Can you work these out from the model? Positions are in its coordinate system, mm. A direction names the side the tool comes from. Round coordinates to 2 decimals unless told otherwise and drop trailing zeros. Order: outer loops, then holes, each group sorted by start corner. A loop starts at its lowest first (then second) coordinate and runs counter-clockwise, first axis right, second up. Notation, with made-up numbers: (72, 6) -> (84, 6) arc R24 ccw to (84, 27) -> close; hole circle Ø7 at (-9.5, -12.5). An arc over 180 degrees is marked (long way). One line per item, written item: value.
```python
from build123d import *

# Parameters (mm, degrees)
F1_R     = 3
F2_DEPTH = 25
F0_R     = 4
F3_DEPTH = 14
F4_R     = 4
F4_R_2   = 3
F5_DEPTH = 11
F7_D     = 4


with BuildPart() as f2:
    # F1 (on Front) → F2 (new body)
    with BuildSketch(Plane.XZ):
        Circle(F1_R)
    extrude(amount=F2_DEPTH)

    # F0 (on Front) → F3 (join)
    with BuildSketch(Plane.XZ):
        Circle(F0_R)
    extrude(amount=F3_DEPTH)

    # F4 (on face) → F5 (cut)
    with BuildSketch(Plane(origin=(0, 0, 0), x_dir=(-1, 0, 0), z_dir=(0, 1, 0))):
        Circle(F4_R)
        Circle(F4_R_2, mode=Mode.SUBTRACT)
    extrude(amount=-F5_DEPTH, mode=Mode.SUBTRACT)

    # F7 (through all)
    with Locations(Plane(origin=(0, 0, 0), x_dir=(-1, 0, 0), z_dir=(0, 1, 0))):
        with Locations((0, 0)):
            Hole(F7_D / 2)


solid = f2.part
```
Q1. I want a section at A-A on x = 0. List the corners of the cut face in (y, z) for me.
Answers below:
outline: (-25, -3) -> (-14, -3) -> (-14, -4) -> (-11, -4) -> (-11, -3) -> (0, -3) -> (0, -2) -> (-25, -2) -> close; (-25, 2) -> (0, 2) -> (0, 3) -> (-11, 3) -> (-11, 4) -> (-14, 4) -> (-14, 3) -> (-25, 3) -> close
Q2. On a 3-axis mill with a long thin cutter (end or side, diameter ignored), from which of +Z, -Z, +X, -X, +Y, -Y can I reach the whole of each face in a straight line? I mean faces 4 (the face through (-1, -11, 3)), 5 (the face through (1, -25, -2)). Say none if no direction works.
Answers below:
face 4: +Y
face 5: +Z, -Z, +X, -X, -Y
Q3. I want a section at B-B on z = 0. List the corners of the cut face in (x, y) for me.
Answers below:
outline: (-4, -14) -> (-3, -14) -> (-3, -25) -> (-2, -25) -> (-2, 0) -> (-3, 0) -> (-3, -11) -> (-4, -11) -> close; (2, -25) -> (3, -25) -> (3, -14) -> (4, -14) -> (4, -11) -> (3, -11) -> (3, 0) -> (2, 0) -> close
Q4. I want a section at C-C on y = -6. List the corners of the cut face in (x, z) for me.
Answers below:
outline: circle Ø6 at (0, 0); hole circle Ø4 at (0, 0)
Q5. Will these pins go through, and if not, where does the flat tip stop? pin 1 Ø1 at (x, y) = (-1.5, -12) entering from +Z; pin 2 Ø3 at (x, z) = (0, 0) entering from -Y; pin 3 Ø1 at (x, y) = (3, -21.5) entering from +Z; pin 4 Ø1 at (x, y) = (1.5, -21) entering from -Z.
Answers below:
pin 1: z = 3.87
pin 2: through
pin 3: z = 1.66
pin 4: z = -2.83
Q6. I want a section at D-D on x = 2.75. List the corners of the cut face in (y, z) for me.
Answers below:
outline: (-25, -1.2) -> (-14, -1.2) -> (-14, -2.9) -> (-11, -2.9) -> (-11, -1.2) -> (0, -1.2) -> (0, 1.2) -> (-11, 1.2) -> (-11, 2.9) -> (-14, 2.9) -> (-14, 1.2) -> (-25, 1.2) -> close
Q7. Please list where these lines run through material, in increasing order: line 1 along Y through (x, z) = (2.25, 3.25); line 2 along Z through (x, y) = (0, -13.5); line 3 along Z through (x, y) = (0, -15).
Answers below:
line 1: -14 to -11
line 2: -4 to -2, 2 to 4
line 3: -3 to -2, 2 to 3
Q8. We'd pull the mould along Z, two halves only. Please class faces 1 (the face through (-3, -19, 0)), 2 (the face through (0, -13, -2)), 3 (the face through (1, -14, 3)): released by +Z, released by -Z, zero draft, split by the parting line, or undercut.
Answers below:
face 1: split by the parting line
face 2: undercut
face 3: zero draft
